from build123d import *

# Parameters (mm, degrees)
RESSALTO_EXTRUS_O1_DEPTH   = 13.9
FILETE1_R                  = 6
CORTE_EXTRUS_O1_DEPTH      = 13.9
FILETE2_R                  = 1.2
CORTE_EXTRUS_O2_DEPTH      = 18.866728856
CORTE_EXTRUS_O2_DEPTH_BACK = 18.866728856
ESBO_O3_W                  = 2
ESBO_O3_H                  = 20.053518914


with BuildPart() as part:
    # Esboço1 → Ressalto-extrusão1 (new body)
    with BuildSketch(Plane(origin=(0, 0, 0), x_dir=(0, 0, -1), z_dir=(1, 0, 0))):
        with BuildLine():
            ThreePointArc((-3.633180425, 4.9), (-1.913112647, 5.792236183), (0, 6.1))
            ThreePointArc((0, 6.1), (1.913112647, 5.792236183), (3.633180425, 4.9))
            ThreePointArc((3.633180425, 4.9), (5.448504409, 2.742954557), (6.1, 0))
            Line((6.1, 0), (10, 0))
            Line((10, 0), (10, 3))
            Line((10, 3), (6, 3))
            Line((6, 3), (6, 8.1))
            Line((6, 8.1), (-6, 8.1))
            Line((-6, 8.1), (-6, 3))
            Line((-6, 3), (-10, 3))
            Line((-10, 3), (-10, 0))
            Line((-10, 0), (-6.1, 0))
            ThreePointArc((-6.1, 0), (-5.448504409, 2.742954557), (-3.633180425, 4.9))
        make_face()
        with BuildLine():
            ThreePointArc((3.633180425, 4.9), (1.913112647, 5.792236183), (0, 6.1))
            Line((0, 6.1), (0, 4.9))
            Line((0, 4.9), (3.633180425, 4.9))
        make_face()
        with BuildLine():
            Line((0, 4.9), (0, 6.1))
            ThreePointArc((0, 6.1), (-1.913112647, 5.792236183), (-3.633180425, 4.9))
            Line((-3.633180425, 4.9), (0, 4.9))
        make_face()
    extrude(amount=RESSALTO_EXTRUS_O1_DEPTH)

    # Filete1
    # the kernel refuses this fillet: 6 mm, written as the material it takes off along each edge
    with BuildSketch(Plane(origin=(-14.83028995, 8.1, 6), x_dir=(0, -1, 0), z_dir=(1, 0, 0))) as filete1_piece_1:
        with BuildLine():
            CenterArc((6, 5.93211598), FILETE1_R, 180, 81.373073441)
            Line((0, 5.93211598), (-0.12, 5.93211598))
            Line((-0.12, 5.93211598), (-0.12, 0))
            Line((-0.12, 0), (0, -0.12))
            ThreePointArc((0, -0.12), (2.55, -0.12), (5.082, -0.11864232))
            Line((5.082, -0.11864232), (5.1, 0))
        make_face()
    extrude(amount=43.5605799, mode=Mode.SUBTRACT)
    with BuildSketch(Plane(origin=(-14.83028995, 8.1, -6), x_dir=(0, -1, 0), z_dir=(1, 0, 0))) as filete1_piece_2:
        with BuildLine():
            CenterArc((6, -5.93211598), FILETE1_R, 98.626926559, 81.373073441)
            Line((0, -5.93211598), (-0.12, -5.93211598))
            Line((-0.12, -5.93211598), (-0.12, 0))
            Line((-0.12, 0), (0, 0.12))
            ThreePointArc((0, 0.12), (2.55, 0.12), (5.082, 0.11864232))
            Line((5.082, 0.11864232), (5.1, 0))
        make_face()
    extrude(amount=43.5605799, mode=Mode.SUBTRACT)

    # Esboço2 → Corte-extrusão1 (cut)
    with BuildSketch(Plane(origin=(0, 3, 0), x_dir=(1, 0, 0), z_dir=(0, 1, 0))):
        with BuildLine():
            ThreePointArc((6.95, 9.35), (5.6, 8), (6.95, 6.65))
            Line((6.95, 6.65), (6.95, 9.35))
        make_face()
        with BuildLine():
            Line((6.95, 9.35), (6.95, 6.65))
            ThreePointArc((6.95, 6.65), (7.904594155, 7.045405845), (8.3, 8))
            ThreePointArc((8.3, 8), (7.904594155, 8.954594155), (6.95, 9.35))
        make_face()
        with BuildLine():
            ThreePointArc((8.3, -8), (7.904594155, -7.045405845), (6.95, -6.65))
            Line((6.95, -6.65), (6.95, -9.35))
            ThreePointArc((6.95, -9.35), (7.904594155, -8.954594155), (8.3, -8))
        make_face()
        with BuildLine():
            Line((6.95, -9.35), (6.95, -6.65))
            ThreePointArc((6.95, -6.65), (5.6, -8), (6.95, -9.35))
        make_face()
    extrude(amount=-CORTE_EXTRUS_O1_DEPTH, mode=Mode.SUBTRACT)

    # Filete2
    filete2_edges = [part.edges().sort_by_distance(p)[0] for p in [
        (6.95, 4.9, -3.633180425),
        (6.95, 4.9, 3.633180425),
    ]]
    fillet(filete2_edges, radius=FILETE2_R)

    # Esboço3 → Corte-extrusão2 (cut, two sides: drawn at the far end of the back side and taken through both)
    with BuildSketch(Plane(origin=(0, 3, 0), x_dir=(1, 0, 0), z_dir=(0, 1, 0)).offset(-CORTE_EXTRUS_O2_DEPTH_BACK)):
        with Locations((1, -0.026759457)):
            Rectangle(ESBO_O3_W, ESBO_O3_H)
    extrude(amount=CORTE_EXTRUS_O2_DEPTH + CORTE_EXTRUS_O2_DEPTH_BACK, mode=Mode.SUBTRACT)


solid = part.part
Input: part model. Units: mm. Frame: model coordinates. A direction names the side the tool comes from. Give positions to 0.01 mm unless a question says otherwise; leave off trailing zeros. Write each loop counter-clockwise with the first axis right and the second up, starting at its lowest first coordinate (ties: lowest second). Pieces come first, ordered by that corner, then holes.
Q1. Material intervals for probe 1 along Z at (x, y) = (7.75, 1.25); probe 2 along Y at (x, z) = (6.75, -6.5); probe 3 along Z at (x, y) = (11.5, 4.25), sorted ascending.
Q2. Set-up query: faces 4 (the face through (9, 3, -8)), 5 (the face through (9, 3, 8)), 6 (the face through (9, 0, -8)), 7 (the face through (7.867, 2.564, -5.535)), 8 (the face through (8, 2, 10)). Return all of +Z, -Z, +X, -X, +Y, -Y with unobstructed straight access to the full face (end or side cutting, diameter ignored); none if empty.
Q3. Section B-B, the plane y = 4.25. Output: boundary loops of the cut face in (x, z).
Q4. Pull-direction query (Z, two-part tool) for faces 1 (the face through (7.87, 6.69, 3.93)), 2 (the face through (8, 1, -10)), 3 (the face through (7.867, 2.498, 5.565)); classes: pulls with the +Z half, pulls with the -Z half, needs draft (parallel to the pull), parting line crosses it, or undercut.
Q5. Section A-A, the plane y = 1. Output: boundary loops of the cut face in (x, z), plus the area to 3 significant figures.
Q6. First-contact query: P1, Ø5, axis at x = 10.5, z = -6, coming from the +Y side; P2, Ø4, axis at y = 7, z = 5.5, coming from the +X side; P3, Ø1.5, axis at x = 7, y = 4.5, coming from the +Z side; P4, Ø1, axis at x = 7.5, z = 3, coming from the -Y side. Flat tips, straight axial feed; report the tip coordinate or a pass-through.
Q7. Section D-D, the plane x = 8.5. Output: boundary loops of the cut face in (y, z), plus the area to 3 significant figures.
Q8. Section C-C, the plane z = -8.5. Output: boundary loops of the cut face in (x, y), plus the area to 3 significant figures.
Filled in:
1. probe 1: z = -10 to -9.09, -6.91 to -5.97, 5.97 to 6.91, 9.09 to 10
1. probe 2: y = 0 to 3
1. probe 3: z = -5.67 to -4.38, 4.38 to 5.67
2. face 4: -Z, +X, -X, +Y
2. face 5: +Z, +X, -X, +Y
2. face 6: +Z, -Z, +X, -X, -Y
2. face 7: +X, -X, -Y
2. face 8: +Z, +X, -X, +Y, -Y
3. outline: (2, -5.67) - (13.9, -5.67) - (13.9, -4.38) - (2, -4.38) - close; (2, 4.38) - (13.9, 4.38) - (13.9, 5.67) - (2, 5.67) - close
4. face 1: pulls with the +Z half
4. face 2: pulls with the -Z half
4. face 3: undercut
5. outline: (2, -10) - (13.9, -10) - (13.9, -6.02) - (2, -6.02) - close; (2, 6.02) - (13.9, 6.02) - (13.9, 10) - (2, 10) - close; hole circle Ø2.7 at (6.95, -8); hole circle Ø2.7 at (6.95, 8)
5. area: 83.3 mm2
6. P1: stops at y = 7.02
6. P2: stops at x = 13.9
6. P3: stops at z = 5.84
6. P4: stops at y = 4.87
7. outline: (0, -10) - (3, -10) - (3, -6) arc R6 ccw to (8.1, -0.07) - (8.1, 0.07) arc R6 ccw to (3, 6) - (3, 10) - (0, 10) - (0, 6.1) arc R6.1 cw to (4.61, 4) arc R1.2 cw to (4.9, 3.21) - (4.9, -3.21) arc R1.2 cw to (4.61, -4) arc R6.1 cw to (0, -6.1) - close
7. area: 54.0 mm2
8. outline: (2, 0) - (5.7, 0) - (5.7, 3) - (2, 3) - close; (8.2, 0) - (13.9, 0) - (13.9, 3) - (8.2, 3) - close
8. area: 28.2 mm2
